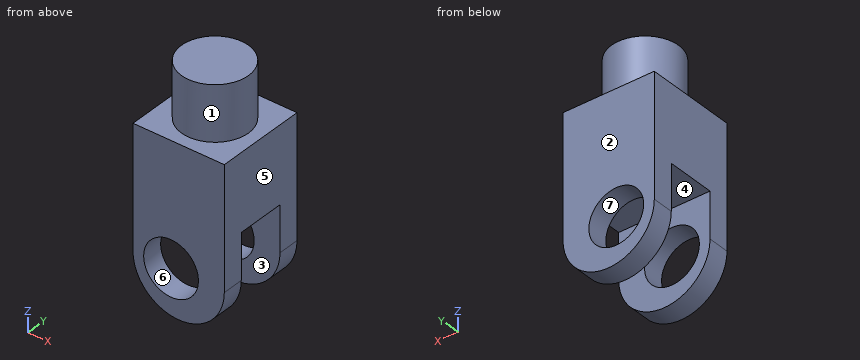
```python
from build123d import *

# Parameters (mm, degrees)
F0_R      = 90
F1_DEPTH  = 180
F2_W      = 300
F2_H      = 300
F3_DEPTH  = 400
F5_DEPTH  = 300
F6_R      = 90
F7_DEPTH  = 300
F8_W      = 160
F8_H      = 300
F9_DEPTH  = 303
F10_R     = 110
F11_DEPTH = 211


with BuildPart() as f1:
    # F0 (on Top) → F1 (new body)
    with BuildSketch(Plane.XY):
        Circle(F0_R)
    extrude(amount=F1_DEPTH)

    # F2 (on face) → F3 (join)
    with BuildSketch(Plane(origin=(0, 0, 0), x_dir=(1, 0, 0), z_dir=(0, 0, -1))):
        Rectangle(F2_W, F2_H)
    extrude(amount=F3_DEPTH)

    # F4 (on face) → F5 (join)
    with BuildSketch(Plane(origin=(0, 150, 0), x_dir=(-1, 0, 0), z_dir=(0, 1, 0))):
        with BuildLine():
            Line((150, -400), (-150, -400))
            ThreePointArc((-150, -400), (0, -550), (150, -400))
        make_face()
    extrude(amount=-F5_DEPTH)

    # F6 (on face) → F7 (cut)
    with BuildSketch(Plane(origin=(0, 150, 0), x_dir=(-1, 0, 0), z_dir=(0, 1, 0))):
        with Locations((25, -400)):
            Circle(F6_R)
    extrude(amount=-F7_DEPTH, mode=Mode.SUBTRACT)

    # F8 (on face) → F9 (cut)
    with BuildSketch(Plane(origin=(-150, 0, 0), x_dir=(0, -1, 0), z_dir=(-1, 0, 0))):
        with Locations((0, -400)):
            Rectangle(F8_W, F8_H)
    extrude(amount=-F9_DEPTH, mode=Mode.SUBTRACT)

    # F10 (on face) → F11 (join)
    with BuildSketch(Plane.XY.offset(180)):
        Circle(F10_R)
    extrude(amount=-F11_DEPTH)


solid = f1.part
```
Can you work these out from the model? Positions are in its coordinate system, mm. Face numbers are marked on the shaded views. A direction names the side the tool comes from. Give positions to 0.01 mm unless a question says otherwise; leave off trailing zeros. Write each loop counter-clockwise with the first axis right and the second up, starting at its lowest first coordinate (ties: lowest second). Pieces come first, ordered by that corner, then holes. Notation, with made-up numbers: (89.25, 63.5) -> (102.25, 63.5) arc R20 ccw to (102.25, 90.5) -> close; hole circle Ø4 at (15.25, 82). An arc over 180 degrees is marked (long way). Write item = value, one per line.
(1) I'm going to push flat-ended pins straight in: P1, Ø6, axis at x = -70, y = -39, coming from the -Z side; P2, Ø3, axis at x = -65, z = 39, coming from the +Y side; P3, Ø5, axis at x = -4, y = -119, coming from the +Z side. Where does each tip first touch, or does it pass through?
Worked out:
P1 = -250
P2 = 89.82
P3 = 0
(2) For the marked faces 1, 2 and 3, which set-ups out of +Z, -Z, +X, -X, +Y, -Y let a thin tool reach every point of the face, with its end or its side?
Worked out:
face_1 = +Z
face_2 = +Z, -Z, +X, -X, +Y
face_3 = -Z, +X, -X
(3) Suppose I cut it at B-B on z = -341. Write out the boundary of the cut face in (x, y), then the cut area to 3 significant figures.
Worked out:
outline = (-150, -150) -> (-92.96, -150) -> (-92.96, -80) -> (-150, -80) -> close; (-150, 80) -> (-92.96, 80) -> (-92.96, 150) -> (-150, 150) -> close; (42.96, -150) -> (150, -150) -> (150, -80) -> (42.96, -80) -> close; (42.96, 80) -> (150, 80) -> (150, 150) -> (42.96, 150) -> close
area = 23,000 mm^2
(4) Thinking about a two-plate mould opening in X: for the marked faces 4, 5, 6 and 7, which applies, released by +X, released by -X, zero draft, split by the parting line, or undercut?
Worked out:
face_4 = zero draft
face_5 = released by +X
face_6 = undercut
face_7 = undercut
(5) Suppose I cut it at A-A on x = 0. Write out the boundary of the cut face in (y, z).
Worked out:
outline = (-150, -550) -> (-80, -550) -> (-80, -486.46) -> (-150, -486.46) -> close; (-150, -313.54) -> (-80, -313.54) -> (-80, -250) -> (80, -250) -> (80, -313.54) -> (150, -313.54) -> (150, 0) -> (110, 0) -> (110, 180) -> (-110, 180) -> (-110, 0) -> (-150, 0) -> close; (80, -550) -> (150, -550) -> (150, -486.46) -> (80, -486.46) -> close
(6) Suppose I cut it at D-D on y = -90. Write out the boundary of the cut face in (x, z).
Worked out:
outline = (-150, -400) arc R150 ccw to (150, -400) -> (150, 0) -> (63.25, 0) -> (63.25, 180) -> (-63.25, 180) -> (-63.25, 0) -> (-150, 0) -> close; hole circle Ø180 at (-25, -400)
(7) Suppose I cut it at C-C on y = 0. Write out the boundary of the cut face in (x, z), then the cut area to 3 significant figures.
Worked out:
outline = (-150, -250) -> (150, -250) -> (150, 0) -> (110, 0) -> (110, 180) -> (-110, 180) -> (-110, 0) -> (-150, 0) -> close
area = 115,000 mm^2
(8) I need wall thicknesses on probe 1 along Y at (x, z) = (91.5, -497.5); probe 2 along Z at (x, y) = (-118.5, 36); probe 3 along Z at (x, y) = (-14.5, -35). Which ranges of each line are inside material? Lowest first, please. Write a range as from..to.
Worked out:
probe_1 = -150..-80, 80..150
probe_2 = -250..0
probe_3 = -250..180
